The listing builds one solid part. Answer for the finished solid, in the listing's coordinates (mm). Coordinates: 2 decimals unless noted, no trailing zeros. Order: outer loops, then holes, each group sorted by start corner. A loop starts at its lowest first (then second) coordinate and runs counter-clockwise, first axis right, second up. Notation, with made-up numbers: (-23, -27) -> (-10, -27) arc R7 ccw to (-10, -15) -> close; hole circle Ø11 at (67.25, 3.25). An arc over 180 degrees is marked (long way). One line per question, with ' | ' between items.
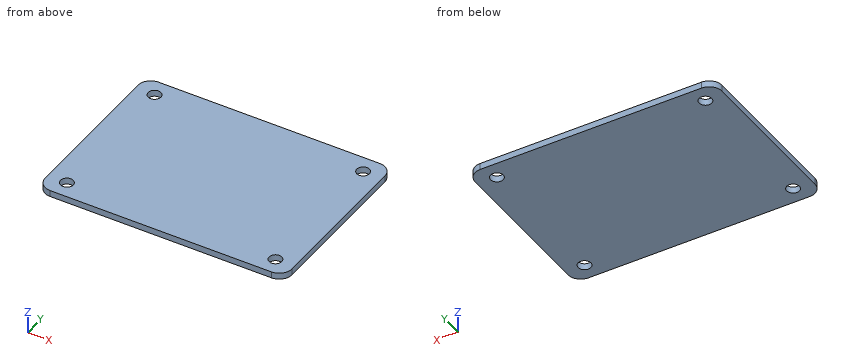
from build123d import *

# Parameters (mm, degrees)
SKETCH_1_W          = 58
SKETCH_1_H          = 42
EXTRUDE_1_DEPTH     = 1.5
SKETCH_2_R          = 1.5
CUT_EXTRUDE_1_DEPTH = 1.5
FILLET_1_R          = 3


with BuildPart() as part:
    # 草图1 → 凸台-拉伸1 (new body)
    with BuildSketch(Plane.XY):
        Rectangle(SKETCH_1_W, SKETCH_1_H)
    extrude(amount=EXTRUDE_1_DEPTH)

    # 草图2 → 切除-拉伸1 (cut)
    with BuildSketch(Plane.XY.offset(1.5)):
        with Locations((-24.5, 17)):
            Circle(SKETCH_2_R)
        with Locations((-24.5, -17)):
            Circle(SKETCH_2_R)
        with Locations((24.5, -17)):
            Circle(SKETCH_2_R)
        with Locations((24.5, 17)):
            Circle(SKETCH_2_R)
    extrude(amount=-CUT_EXTRUDE_1_DEPTH, mode=Mode.SUBTRACT)

    # 圆角1
    fillet_1_edges = [part.edges().sort_by_distance(p)[0] for p in [
        (29, -21, 0.75),
        (-29, -21, 0.75),
        (-29, 21, 0.75),
        (29, 21, 0.75),
    ]]
    fillet(fillet_1_edges, radius=FILLET_1_R)


solid = part.part
Item 1: Section B-B, the plane y = 17 is taken. Give the vertices of the cut face in (x, z).
Computed values:
outline: (-29, 0) -> (-26, 0) -> (-26, 1.5) -> (-29, 1.5) -> close; (-23, 0) -> (23, 0) -> (23, 1.5) -> (-23, 1.5) -> close; (26, 0) -> (29, 0) -> (29, 1.5) -> (26, 1.5) -> close
Item 2: Find the intervals of material crossed by L1, parallel to Y at x = 24.5, z = 0.45; L2, parallel to X at y = -19, z = 0.65, in increasing order.
Computed values:
L1: y = -21 to -18.5, -15.5 to 15.5, 18.5 to 21 | L2: x = -28.83 to 28.83
Item 3: Section A-A, the plane x = 24.5 is taken. Give the vertices of the cut face in (y, z), plus the area to 3 significant figures.
Computed values:
outline: (-21, 0) -> (-18.5, 0) -> (-18.5, 1.5) -> (-21, 1.5) -> close; (-15.5, 0) -> (15.5, 0) -> (15.5, 1.5) -> (-15.5, 1.5) -> close; (18.5, 0) -> (21, 0) -> (21, 1.5) -> (18.5, 1.5) -> close | area: 54.0 mm^2
Item 4: This flat-tipped pin is pushed along its axis until it touches: pin 1 Ø4 at (x, y) = (-24.5, 17) entering from -Z. Where does it stop, or does it pass through?
Computed values:
pin 1: stops at z = 0
